from build123d import *

# Parameters (mm, degrees)
SKETCH1_R           = 16.5
SKETCH1_R_2         = 2.075
BOSS_EXTRUDE1_DEPTH = 2.5


with BuildPart() as part:
    # Sketch1 → Boss-Extrude1 (new body)
    with BuildSketch(Plane(origin=(0, 0, 0), x_dir=(1, 0, 0), z_dir=(0, 1, 0))):
        with Locations(Location((0, 0, 0), (0, 0, 270))):
            Circle(SKETCH1_R)
        with Locations(Location((0, 0, 0), (0, 0, 270))):
            Circle(SKETCH1_R_2, mode=Mode.SUBTRACT)
        with BuildLine():
            Line((-3.5, 0), (-15, 0))
            ThreePointArc((-15, 0), (-4.877508592, -14.1848479), (11.827987991, -9.224895668))
            Line((11.827987991, -9.224895668), (1.403459084, -3.206291097))
            ThreePointArc((1.403459084, -3.206291097), (-1.915449452, -2.92934351), (-3.5, 0))
        make_face(mode=Mode.SUBTRACT)
        with BuildLine():
            Line((-11.827987991, 9.224895668), (-1.403459084, 3.206291097))
            ThreePointArc((-1.403459084, 3.206291097), (1.915449452, 2.92934351), (3.5, 0))
            Line((3.5, 0), (15, 0))
            ThreePointArc((15, 0), (4.877508592, 14.1848479), (-11.827987991, 9.224895668))
        make_face(mode=Mode.SUBTRACT)
    extrude(amount=BOSS_EXTRUDE1_DEPTH)


solid = part.part
CAD build for the part. Positions are in the model's coordinates, mm. A direction names the side the tool comes from. Give positions to 0.01 mm unless a question says otherwise; leave off trailing zeros. Write each loop counter-clockwise with the first axis right and the second up, starting at its lowest first coordinate (ties: lowest second). Pieces come first, ordered by that corner, then holes. Notation, with made-up numbers: (23, 0.25) - (43, 0.25) arc R29 cw to (43, 23.25) - close; hole circle Ø9 at (56.25, -18). An arc over 180 degrees is marked (long way). Answer as CSV lines item,"result".
Q1. Drill centre lines: line 1 (Z direction, x = 1, y = 2.05); line 2 (X direction, y = 0.85, z = 1); line 3 (X direction, y = 2.25, z = -1.5). Where is each one in solid material? Low to high. Write a range as from..to.
Result set:
line 1,"-16.47..-14.97, -3.35..-1.82, 1.82..3.35, 14.97..16.47"
line 2,"-16.47..-14.97, -3.35..-1.82, 1.82..16.47"
line 3,"-16.43..-1.43, 1.43..3.16, 14.92..16.43"
Q2. Band-saw the part on B-B (y = 1.9). Give the cut face in (x, z) (3 decimals), and give its area (3 significant figures).
Result set:
outline,"circle Ø33 at (0, 0); hole (-15, 0) - (-3.5, 0) arc R3.5 cw to (1.403, 3.206) - (11.828, 9.225) arc R15 ccw to start; hole (-11.828, -9.225) arc R15 ccw to (15, 0) - (3.5, 0) arc R3.5 cw to (-1.403, -3.206) - close; hole circle Ø4.15 at (0, 0)"
area,"333 mm²"
Q3. Band-saw the part on A-A (x = 0). Give the cut face in (y, z) (3 decimals), and give its area (3 significant figures).
Result set:
outline,"(0, -16.5) - (2.5, -16.5) - (2.5, -15) - (0, -15) - close; (0, -3.5) - (2.5, -3.5) - (2.5, -2.075) - (0, -2.075) - close; (0, 2.075) - (2.5, 2.075) - (2.5, 3.5) - (0, 3.5) - close; (0, 15) - (2.5, 15) - (2.5, 16.5) - (0, 16.5) - close"
area,"14.6 mm²"
Q4. Band-saw the part on D-D (x = 13). Give the cut face in (y, z), and give its area (3 significant figures).
Result set:
outline,"(0, -10.16) - (2.5, -10.16) - (2.5, -7.48) - (0, -7.48) - close; (0, 0) - (2.5, 0) - (2.5, 10.16) - (0, 10.16) - close"
area,"32.1 mm²"
Q5. Pull direction X, two halves, no side cores. Call faces 1 (the face through (6.69, 1.23, 6.26)), 2 (the face through (0.1, 0, 2.4)), 3 (the face through (-16.108, 1.232, -3.577)): released by +X, released by -X, zero draft, split by the parting line, or undercut.
Result set:
face 1,"undercut"
face 2,"zero draft"
face 3,"split by the parting line"
Q6. Flat gauge pins, fed straight in: pin 1 Ø1.2 at (x, y) = (10, 1) entering from -Z; pin 2 Ø1 at (y, z) = (2, -8.5) entering from +X; pin 3 Ø12 at (x, z) = (3, -5.5) entering from -Y; pin 4 Ø1 at (x, y) = (11.5, 1.5) entering from -Z. Where does each tip first touch, or does it go through?
Result set:
pin 1,"z = -13.56"
pin 2,"x = 14.43"
pin 3,"y = 0"
pin 4,"z = -12.3"
Q7. Band-saw the part on C-C (z = 5.5). Give the cut face in (x, y), and give its area (3 significant figures).
Result set:
outline,"(-15.56, 0) - (-13.96, 0) - (-13.96, 2.5) - (-15.56, 2.5) - close; (5.38, 0) - (15.56, 0) - (15.56, 2.5) - (5.38, 2.5) - close"
area,"29.5 mm²"
Q8. 3-axis set-ups, long thin cutter, end or side, ignore diameter. For faces 4 (the face through (-5.12, 1.23, 14.1)), 5 (the face through (0.1, 2.5, 2.4)): which of +Z, -Z, +X, -X, +Y, -Y reach the whole face in a straight line?
Result set:
face 4,"+Y, -Y"
face 5,"+Z, -Z, +X, -X, +Y"
